Source: three-view drawing plus pictorial views. Frame: mm from the lowest corner of the part. Coordinates: 2 decimals unless noted, no trailing zeros. Write each loop counter-clockwise with the first axis right and the second up, starting at its lowest first coordinate (ties: lowest second). Pieces come first, ordered by that corner, then holes. Notation, with made-up numbers: (50.5, 85.25) - (73.5, 85.25) arc R8 cw to (73.5, 98.25) - close; hole circle Ø8 at (50, 33). An arc over 180 degrees is marked (long way). One line per item, written item: value.
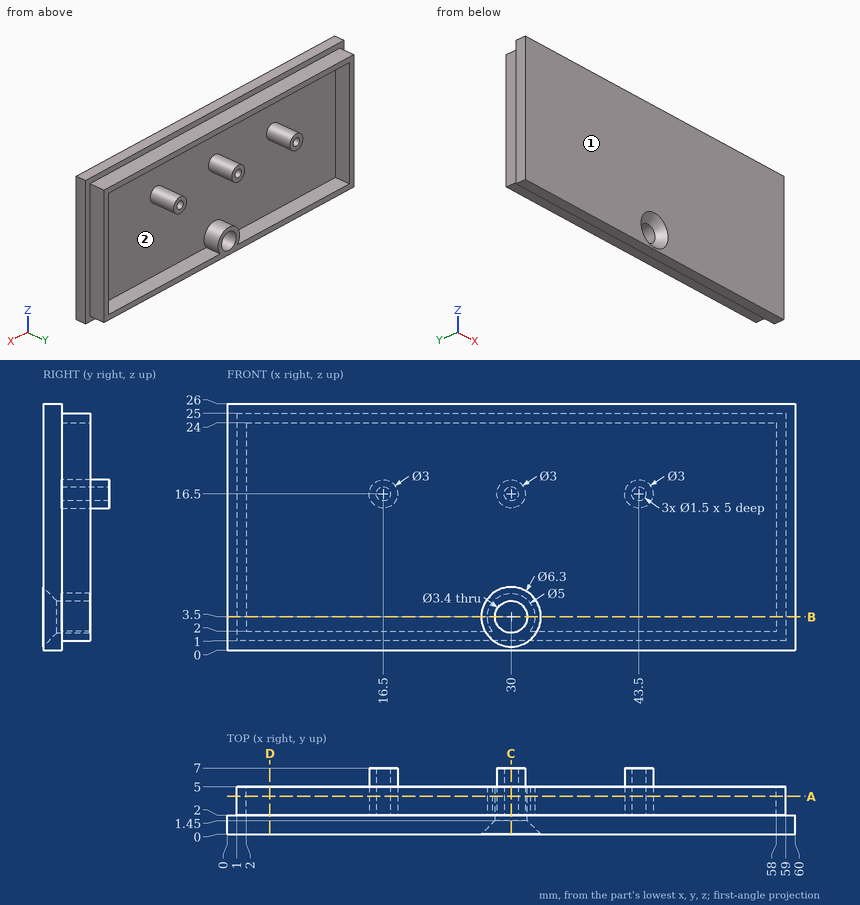
1) Material intervals for line 1 (X direction, y = 5.65, z = 16.5); line 2 (X direction, y = 3.2, z = 3.5); line 3 (Z direction, x = 8, y = 4), sorted ascending.
Values found:
line 1: 15 to 15.75, 17.25 to 18, 28.5 to 29.25, 30.75 to 31.5, 42 to 42.75, 44.25 to 45
line 2: 1 to 2, 27.5 to 28.3, 31.7 to 32.5, 58 to 59
line 3: 1 to 2, 24 to 25
2) Draft query along Z for the marked faces 1 and 2. Return one class per face: released by +Z, released by -Z, zero draft, split by the parting line, or undercut.
Values found:
face 1: zero draft
face 2: undercut
3) Section query D-D on x = 4.5. Output: boundary loops of the cut face in (y, z), then the cut area to 3 significant figures.
Values found:
outline: (0, 0) - (2, 0) - (2, 1) - (5, 1) - (5, 2) - (2, 2) - (2, 24) - (5, 24) - (5, 25) - (2, 25) - (2, 26) - (0, 26) - close
area: 58.0 mm2
4) Section query C-C on x = 30. Output: boundary loops of the cut face in (y, z).
Values found:
outline: (0, 0) - (2, 0) - (2, 1) - (5, 1) - (5, 1.8) - (1.45, 1.8) - (0, 0.35) - close; (0, 6.65) - (1.45, 5.2) - (5, 5.2) - (5, 6) - (2, 6) - (2, 15) - (7, 15) - (7, 15.75) - (2, 15.75) - (2, 17.25) - (7, 17.25) - (7, 18) - (2, 18) - (2, 24) - (5, 24) - (5, 25) - (2, 25) - (2, 26) - (0, 26) - close
5) Section query A-A on y = 4. State how many separate pieces and enclosed holes the cut face has, then the cut area to 3 significant figures.
Values found:
separate pieces: 4
enclosed holes: 5
area: 184 mm2
6) Section query B-B on z = 3.5. Output: boundary loops of the cut face in (x, y), then the cut area to 3 significant figures.
Values found:
outline: (0, 0) - (26.85, 0) - (28.3, 1.45) - (28.3, 5) - (27.5, 5) - (27.5, 2) - (2, 2) - (2, 5) - (1, 5) - (1, 2) - (0, 2) - close; (31.7, 1.45) - (33.15, 0) - (60, 0) - (60, 2) - (59, 2) - (59, 5) - (58, 5) - (58, 2) - (32.5, 2) - (32.5, 5) - (31.7, 5) - close
area: 122 mm2
7) Contact query for flat-ended pins moving along their axis: P1, Ø1, axis at x = 7, y = 5, coming from the +Z side; P2, Ø3, axis at x = 32.5, y = 5, coming from the -Z side; P3, Ø12, axis at x = 11, z = 11, coming from the +Y side. Output: stop coordinate, or through.
Values found:
P1: z = 25
P2: z = 1
P3: y = 2
